from build123d import *

# Parameters (mm, degrees)
SKETCH1_W               = 190
SKETCH1_H               = 50
BOSS_EXTRUDE1_DEPTH     = 120
SHELL1_T                = 5
SKETCH2_R               = 1.7
CUT_EXTRUDE1_DEPTH      = 168.705098312
CUT_EXTRUDE1_DEPTH_BACK = 168.705098312
SKETCH3_R               = 6.75
CUT_EXTRUDE2_DEPTH      = 168.705098312
CUT_EXTRUDE2_DEPTH_BACK = 168.705098312


with BuildPart() as part:
    # Sketch1 → Boss-Extrude1 (new, symmetric)
    with BuildSketch(Plane.XY):
        with Locations((0, 25)):
            Rectangle(SKETCH1_W, SKETCH1_H)
    extrude(amount=BOSS_EXTRUDE1_DEPTH, both=True)

    # Shell1
    shell1_openings = [part.faces().sort_by_distance(p)[0] for p in [
        (0, 50, 0),
    ]]
    offset(amount=SHELL1_T, openings=shell1_openings, kind=Kind.INTERSECTION)

    # Sketch2 → Cut-Extrude1 (cut, two sides)
    with BuildSketch(Plane(origin=(0, 0, 0), x_dir=(1, 0, 0), z_dir=(0, 1, 0))) as cut_extrude1_sk:
        with Locations(Location((-12.5, 70, 0), (0, 0, 180))):
            Circle(SKETCH2_R)
        with Locations(Location((-37.5, 30, 0), (0, 0, 180))):
            Circle(SKETCH2_R)
        with Locations(Location((-62.5, 30, 0), (0, 0, 180))):
            Circle(SKETCH2_R)
        with Locations(Location((-82.5, 35, 0), (0, 0, 180))):
            Circle(SKETCH2_R)
        with Locations(Location((82.5, 35, 0), (0, 0, 180))):
            Circle(SKETCH2_R)
        with Locations(Location((62.5, 30, 0), (0, 0, 180))):
            Circle(SKETCH2_R)
        with Locations(Location((37.5, 30, 0), (0, 0, 180))):
            Circle(SKETCH2_R)
        with Locations(Location((12.5, 70, 0), (0, 0, 180))):
            Circle(SKETCH2_R)
        with Locations(Location((12.5, -70, 0), (0, 0, 180))):
            Circle(SKETCH2_R)
        with Locations(Location((37.5, -30, 0), (0, 0, 180))):
            Circle(SKETCH2_R)
        with Locations(Location((62.5, -30, 0), (0, 0, 180))):
            Circle(SKETCH2_R)
        with Locations(Location((82.5, -35, 0), (0, 0, 180))):
            Circle(SKETCH2_R)
        with Locations(Location((-82.5, -35, 0), (0, 0, 180))):
            Circle(SKETCH2_R)
        with Locations(Location((-62.5, -30, 0), (0, 0, 180))):
            Circle(SKETCH2_R)
        with Locations(Location((-37.5, -30, 0), (0, 0, 180))):
            Circle(SKETCH2_R)
        with Locations(Location((-12.5, -70, 0), (0, 0, 180))):
            Circle(SKETCH2_R)
    extrude(amount=CUT_EXTRUDE1_DEPTH, mode=Mode.SUBTRACT)
    extrude(cut_extrude1_sk.sketch, amount=-CUT_EXTRUDE1_DEPTH_BACK, mode=Mode.SUBTRACT)

    # Sketch3 → Cut-Extrude2 (cut, two sides)
    with BuildSketch(Plane(origin=(0, 0, 0), x_dir=(0, 0, -1), z_dir=(1, 0, 0))) as cut_extrude2_sk:
        with Locations((0, 15)):
            Circle(SKETCH3_R)
    extrude(amount=CUT_EXTRUDE2_DEPTH, mode=Mode.SUBTRACT)
    extrude(cut_extrude2_sk.sketch, amount=-CUT_EXTRUDE2_DEPTH_BACK, mode=Mode.SUBTRACT)


solid = part.part
Design review of the part built by this model. Coordinates are the model's own, in mm. A direction names the side the tool comes from. Give positions to 0.01 mm unless a question says otherwise; leave off trailing zeros. Loops run counter-clockwise (first coordinate to the right, second up) from the corner with the lowest first, then second, coordinate; pieces in that order, holes last. Notation, with made-up numbers: M 81,86.25 L 85,86.25 A23 ccw 85,122.25 Z; hole C 24.5,3.25 d7. An arc over 180 degrees is marked long. Answer as a JSON object with one key per item and string values.
Item 1: We need section B-B (z = -104.5). State the section outline as (x, y) points.
Output values:
{"outline": "M -100,-5 L 100,-5 L 100,50 L 95,50 L 95,0 L -95,0 L -95,50 L -100,50 Z"}
Item 2: Machinability: for faces 4 (the face through (0, 50, 121)), 5 (the face through (-95, 25, 2)), which of the approach directions +Z, -Z, +X, -X, +Y, -Y give a long, thin tool a straight path to every point of the face, cutting with its end or side? Answer none if there is none.
Output values:
{"face 4": "+Z, -Z, +X, -X, +Y", "face 5": "+Y"}
Item 3: Mouldability with a two-part tool opening along X and no side actions: class faces 1 (the face through (-97.46, 8.41, 1.46)), 2 (the face through (-100, 22, 2)), 3 (the face through (-1, 0, 2)) as pulls with the +X half, pulls with the -X half, needs draft (parallel to the pull), parting line crosses it, or undercut.
Output values:
{"face 1": "needs draft", "face 2": "pulls with the -X half", "face 3": "undercut"}
Item 4: We need section C-C (x = 73). State the section outline as (y, z) points.
Output values:
{"outline": "M -5,-125 L 50,-125 L 50,-120 L 0,-120 L 0,120 L 50,120 L 50,125 L -5,125 Z"}
Item 5: We need section D-D (y = 35.5). State the section outline as (x, z) points, and give its area (3 significant figures).
Output values:
{"outline": "M -100,-125 L 100,-125 L 100,125 L -100,125 Z; hole M -95,-120 L 95,-120 L 95,120 L -95,120 Z", "area": "4,400 mm2"}
Item 6: Wall thickness on line 1 along Z through (x, y) = (62.5, -1.6); line 2 along Z through (x, y) = (19.5, 48); line 3 along Z through (x, y) = (97, 15): over which ranges is each line inside the solid? List them lowest first.
Output values:
{"line 1": "z = -125 to -31.7, -28.3 to 28.3, 31.7 to 125", "line 2": "z = -125 to -120, 120 to 125", "line 3": "z = -125 to -6.75, 6.75 to 125"}
Item 7: We need section A-A (y = 15). State the section outline as (x, z) points, and give its area (4 significant figures).
Output values:
{"outline": "M -100,-125 L 100,-125 L 100,-6.75 L 95,-6.75 L 95,-120 L -95,-120 L -95,-6.75 L -100,-6.75 Z; M -100,6.75 L -95,6.75 L -95,120 L 95,120 L 95,6.75 L 100,6.75 L 100,125 L -100,125 Z", "area": "4,265 mm2"}
Item 8: For P1, Ø11, axis at y = 15, z = 0, coming from the -X side; P2, Ø4.5, axis at x = 37.5, z = -30, coming from the +Y side, all flat-tipped, find the tip position at first contact; note any pin that passes through.
Output values:
{"P1": "passes through", "P2": "stops at y = 0"}
